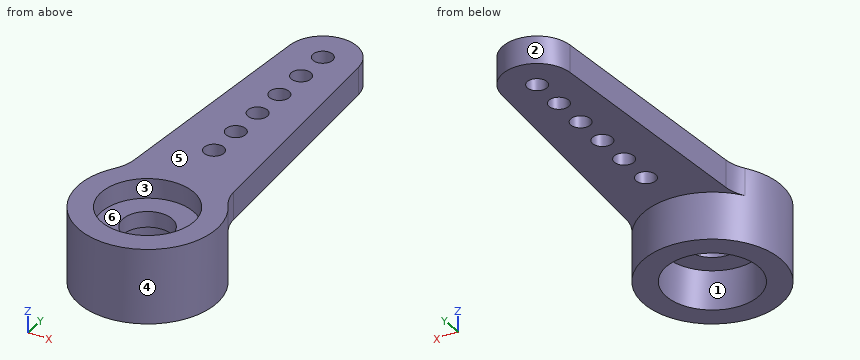
```python
from build123d import *

# Parameters (mm, degrees)
SKIZZE1_R                       = 3.5
SKIZZE1_R_2                     = 1.25
AUFSATZ_LINEAR_AUSTRAGEN1_DEPTH = 3.8
SKIZZE2_R                       = 0.5
AUFSATZ_LINEAR_AUSTRAGEN2_DEPTH = 1.4
SKIZZE3_R                       = 2.35
SCHNITT_LINEAR_AUSTRAGEN1_DEPTH = 1
SCHNITT_LINEAR_START            = -2
SKIZZE4_R                       = 2.35
SCHNITT_LINEAR_AUSTRAGEN2_DEPTH = 2
VERRUNDUNG1_R                   = 2


with BuildPart() as part:
    # Skizze1 → Aufsatz-Linear austragen1 (new body)
    with BuildSketch(Plane.XY):
        with Locations(Location((0, 0, 0), (0, 0, 180))):
            Circle(SKIZZE1_R)
        with Locations(Location((0, 0, 0), (0, 0, 180))):
            Circle(SKIZZE1_R_2, mode=Mode.SUBTRACT)
    extrude(amount=AUFSATZ_LINEAR_AUSTRAGEN1_DEPTH)

    # Skizze2 → Aufsatz-Linear austragen2 (add)
    with BuildSketch(Plane.XY.offset(3.8)):
        with BuildLine():
            Line((2.65, 1.25), (-2.65, 1.25))
            Line((-2.65, 1.25), (-1.746012422, 14.618070409))
            ThreePointArc((-1.746012422, 14.618070409), (0, 16.25), (1.746012422, 14.618070409))
            Line((1.746012422, 14.618070409), (2.65, 1.25))
        make_face()
        with Locations((0, 14.5)):
            Circle(SKIZZE2_R, mode=Mode.SUBTRACT)
        with Locations((0, 12.7)):
            Circle(SKIZZE2_R, mode=Mode.SUBTRACT)
        with Locations((0, 10.9)):
            Circle(SKIZZE2_R, mode=Mode.SUBTRACT)
        with Locations((0, 9.1)):
            Circle(SKIZZE2_R, mode=Mode.SUBTRACT)
        with Locations((0, 7.3)):
            Circle(SKIZZE2_R, mode=Mode.SUBTRACT)
        with Locations((0, 5.5)):
            Circle(SKIZZE2_R, mode=Mode.SUBTRACT)
    extrude(amount=-AUFSATZ_LINEAR_AUSTRAGEN2_DEPTH)

    # Skizze3 → Schnitt-Linear austragen1 (cut)
    with BuildSketch(Plane.XY.offset(3.8)):
        Circle(SKIZZE3_R)
    extrude(amount=-SCHNITT_LINEAR_AUSTRAGEN1_DEPTH, mode=Mode.SUBTRACT)

    # Skizze4 → Schnitt-Linear austragen2 (cut)
    with BuildSketch(Plane(origin=(0, 0, 0), x_dir=(-1, 0, 0), z_dir=(0, 0, -1)).offset(SCHNITT_LINEAR_START)):
        with Locations(Location((0, 0, 0), (0, 0, 180))):
            Circle(SKIZZE4_R)
    extrude(amount=SCHNITT_LINEAR_AUSTRAGEN2_DEPTH, mode=Mode.SUBTRACT)

    # Verrundung1
    verrundung1_edges = [part.edges().sort_by_distance(p)[0] for p in [
        (-2.5741658, 2.371427931, 3.1),
        (2.5741658, 2.371427931, 3.1),
    ]]
    fillet(verrundung1_edges, radius=VERRUNDUNG1_R)


solid = part.part
```
CAD build for the part. Positions are in the model's coordinates, mm. Face numbers are marked on the shaded views. A direction names the side the tool comes from. Give positions to 0.01 mm unless a question says otherwise; leave off trailing zeros. Order: outer loops, then holes, each group sorted by start corner. A loop starts at its lowest first (then second) coordinate and runs counter-clockwise, first axis right, second up. Notation, with made-up numbers: M -31,-15.75 L -20,-15.75 A28 cw -20,12.25 Z; hole C -23,60 d4. An arc over 180 degrees is marked long. Put each result on its own line as item: value. Start each with the question number.
(1) Flat gauge pins, fed straight in: pin 1 Ø2.5 at (x, y) = (0, -0.5) entering from +Z; pin 2 Ø1.5 at (y, z) = (6.5, 3) entering from -X; pin 3 Ø4 at (x, y) = (-0.5, 0.5) entering from -Z. Where does each tip first touch, or does it go through?
(2) Mould opens along Y. For the marked faces 4, 5 and 6 say: +Y half, -Y half, draft (parallel to the pull), parting line (faces both ways), or undercut.
(3) Saw through at D-D, the plane z = 1.5. Write the cut outline in (x, y).
(4) Saw through at C-C, the plane x = 0. Give the number of separate pieces and of enclosed holes in the cut face, then the cut area to 4 significant figures.
(5) Drill centre lines: line 1 along Y through (x, z) = (0, 0.8); line 2 along Z through (x, y) = (0.5, 8.5); line 3 along Y through (x, z) = (1, 1.6). Where is each one in solid material? Low to high.
(6) Saw through at A-A, the plane z = 3.15. Write the cut outline in (x, y), then the cut area to 3 significant figures.
(7) Saw through at B-B, the plane y = 10.9. Write the cut outline in (x, z), then the cut area to 3 significant figures.
(8) Which spindle directions (+Z, -Z, +X, -X, +Y, -Y) get a long thin tool onto all of the face, cutting with end or side? Do the marked faces 1, 2 and 3. Say none if no direction does.
Check result:
1. pin 1: stops at z = 2.8
1. pin 2: stops at x = -2.35
1. pin 3: stops at z = 0
2. face 4: parting line
2. face 5: draft
2. face 6: undercut
3. outline: C 0,0 d7; hole C 0,0 d4.7
4. separate pieces: 8
4. enclosed holes: 0
4. area: 19.95 mm2
5. line 1: y = -3.5 to -2.35, 2.35 to 3.5
5. line 2: z = 2.4 to 3.8
5. line 3: y = -3.35 to -2.13, 2.13 to 3.35
6. outline: M -2.88,1.99 A3.5 ccw long 2.88,1.99 A2 cw 2.53,2.99 L 1.75,14.62 A1.75 ccw -1.75,14.62 L -2.53,2.99 A2 cw Z; hole C 0,0 d4.7; hole C 0,5.5 d1; hole C 0,7.3 d1; hole C 0,9.1 d1; hole C 0,10.9 d1; hole C 0,12.7 d1; hole C 0,14.5 d1
6. area: 69.8 mm2
7. outline: M -2,2.4 L -0.5,2.4 L -0.5,3.8 L -2,3.8 Z; M 0.5,2.4 L 2,2.4 L 2,3.8 L 0.5,3.8 Z
7. area: 4.19 mm2
8. face 1: -Z
8. face 2: +Z, -Z, +Y
8. face 3: +Z
